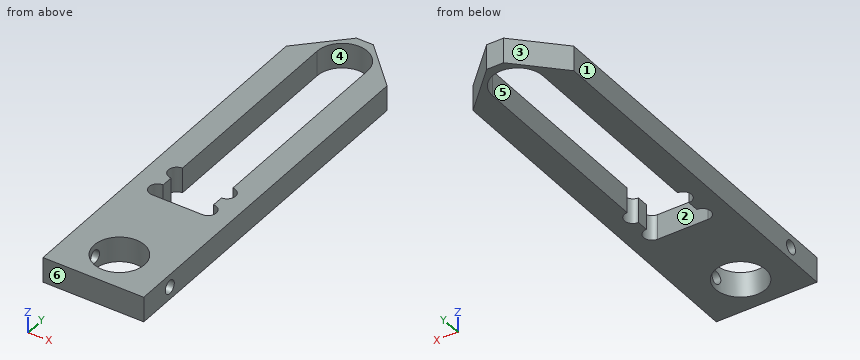
```python
from build123d import *

# Parameters (mm, degrees)
BASE_EXTRUSION_DEPTH    = 15
ESQUISSE2_R             = 15
ENL_V_MAT_EXTRU_1_DEPTH = 15
ENL_V_MAT_EXTRU_2_DEPTH = 15
ESQUISSE4_R             = 4
ENL_V_MAT_EXTRU_3_DEPTH = 248.840674628


with BuildPart() as part:
    # Esquisse1 → Base-Extrusion (new body)
    with BuildSketch(Plane.XY):
        Polygon((0, 215), (25, 240), (35, 240), (60, 215), (60, 0), (0, 0), align=None)
    extrude(amount=BASE_EXTRUSION_DEPTH)

    # Esquisse2 → Enlèv. mat.-Extru.1 (cut)
    with BuildSketch(Plane.XY.offset(15)):
        with Locations((30, 23)):
            Circle(ESQUISSE2_R)
    extrude(amount=-ENL_V_MAT_EXTRU_1_DEPTH, mode=Mode.SUBTRACT)

    # Esquisse3 → Enlèv. mat.-Extru.2 (cut)
    with BuildSketch(Plane.XY.offset(15)):
        with BuildLine():
            Line((45, 91), (45, 84))
            ThreePointArc((45, 84), (50, 79), (45, 74))
            Line((45, 74), (15, 74))
            ThreePointArc((15, 74), (10, 79), (15, 84))
            Line((15, 84), (15, 91))
            ThreePointArc((15, 91), (10, 96), (15, 101))
            Line((15, 101), (15, 220))
            ThreePointArc((15, 220), (30, 235), (45, 220))
            Line((45, 220), (45, 101))
            ThreePointArc((45, 101), (50, 96), (45, 91))
        make_face()
    extrude(amount=-ENL_V_MAT_EXTRU_2_DEPTH, mode=Mode.SUBTRACT)

    # Esquisse4 → Enlèv. mat.-Extru.3 (cut, through all)
    with BuildSketch(Plane.ZY):
        with Locations((7.5, 23)):
            Circle(ESQUISSE4_R)
    extrude(amount=-ENL_V_MAT_EXTRU_3_DEPTH, mode=Mode.SUBTRACT)


solid = part.part
```
For this review, take the finished solid that the model builds, in its own axes (mm). Face numbers are marked on the shaded views. A direction names the side the tool comes from. Give positions to 0.01 mm unless a question says otherwise; leave off trailing zeros. Order: outer loops, then holes, each group sorted by start corner. A loop starts at its lowest first (then second) coordinate and runs counter-clockwise, first axis right, second up.
1) For the marked faces 5 and 6, list the 3-axis set-ups (+Z, -Z, +X, -X, +Y, -Y) from which the entire face can be reached by the end or side of a thin tool; tool diameter is ignored.
2) Take a section at B-B (x = 48). Give the boundary of the cut face in (y, z).
3) Take a section at D-D (x = 39). Give the boundary of the cut face in (y, z), then the cut area to 3 significant figures.
4) Take a section at C-C (y = 23). Give the boundary of the cut face in (x, z), then the cut area to 3 significant figures.
5) Wall thickness on line 1 (Y direction, x = 30, z = 4.25); line 2 (Y direction, x = 25.5, z = 13.5); line 3 (X direction, y = 206.5, z = 3.75): over which ranges is each line inside the solid? List them lowest first.
6) Take a section at A-A (z = 7.5). Give the boundary of the cut face in (x, y).
7) The part is to be moulded in two halves that separate along Y. For the marked faces 1, 2, 3 and 4, say which applies: released by +Y, released by -Y, zero draft, split by the parting line, or undercut.
Derived:
1. face 5: +Z, -Z
1. face 6: +Z, -Z, +X, -X, -Y
2. outline: (0, 0) - (75, 0) - (75, 15) - (0, 15) - close; (83, 0) - (92, 0) - (92, 15) - (83, 15) - close; (100, 0) - (227, 0) - (227, 15) - (100, 15) - close; hole circle Ø8 at (23, 7.5)
3. outline: (0, 0) - (11, 0) - (11, 15) - (0, 15) - close; (35, 0) - (74, 0) - (74, 15) - (35, 15) - close; (232, 0) - (236, 0) - (236, 15) - (232, 15) - close
3. area: 810 mm2
4. outline: (0, 0) - (15, 0) - (15, 3.5) - (0, 3.5) - close; (0, 11.5) - (15, 11.5) - (15, 15) - (0, 15) - close; (45, 0) - (60, 0) - (60, 3.5) - (45, 3.5) - close; (45, 11.5) - (60, 11.5) - (60, 15) - (45, 15) - close
4. area: 210 mm2
5. line 1: y = 0 to 8, 38 to 74, 235 to 240
5. line 2: y = 0 to 8.69, 37.31 to 74, 234.31 to 240
5. line 3: x = 0 to 15, 45 to 60
6. outline: (0, 0) - (60, 0) - (60, 19) - (44.46, 19) arc R15 cw to (15.54, 19) - (0, 19) - close; (0, 27) - (15.54, 27) arc R15 cw to (44.46, 27) - (60, 27) - (60, 215) - (35, 240) - (25, 240) - (0, 215) - close; hole (15, 74) - (45, 74) arc R5 ccw to (45, 84) - (45, 91) arc R5 ccw to (45, 101) - (45, 220) arc R15 ccw to (15, 220) - (15, 101) arc R5 ccw to (15, 91) - (15, 84) arc R5 ccw to start
7. face 1: zero draft
7. face 2: undercut
7. face 3: released by +Y
7. face 4: undercut
